Read the model definition and answer for the solid it produces. Units are mm, in the model's axes. Face numbers are marked on the shaded views. A direction names the side the tool comes from. Coordinates: 2 decimals unless noted, no trailing zeros. Order: outer loops, then holes, each group sorted by start corner. A loop starts at its lowest first (then second) coordinate and runs counter-clockwise, first axis right, second up. Notation, with made-up numbers: M 58,75.25 L 88,75.25 A23 cw 88,108.25 Z; hole C -31,61 d3. An arc over 180 degrees is marked long. Use a Markdown table: item, result. Add a question column.
1) For the marked faces 4, 5, 6, 7 and 8, determine the directions among +Z, -Z, +X, -X, +Y, -Y from which every point of the face is accessible in a straight line to the end or side of a thin tool.
2) Find section C-C on z = -30. Write down the section's boundary in (x, y).
3) The mould has two halves that part along Z. Classify the marked faces 1, 2 and 3: released by +Z, released by -Z, zero draft, split by the parting line, or undercut.
4) Find section D-D on z = -46.9. Write down the section's boundary in (x, y), plus the area to 3 significant figures.
5) Each of these flat-tipped pins is pushed along its axis until it touches: pin 1 Ø2.5 at (x, z) = (9.5, -1.5) entering from -Y; pin 2 Ø1.5 at (x, y) = (4.5, -32.5) entering from -Z; pin 3 Ø2.5 at (y, z) = (2.53, -46.9) entering from -X; pin 4 Ø3 at (x, y) = (4, -26) entering from +Z. Where does it stop, or does it pass through?
6) Find section B-B on y = -23. Write down the section's boundary in (x, z), plus the area to 3 significant figures.
7) Find section A-A on z = -60. Write down the section's boundary in (x, y), plus the area to 3 significant figures.
8) Find the intervals of material crossed by probe 1 along Z at (x, y) = (8.5, -32); probe 2 along Z at (x, y) = (8.5, 1); probe 3 along Y at (x, z) = (9.5, -18), in increasing order. Write a range as [from, to].
from build123d import *

# Parameters (mm, degrees)
SKETCH1_W           = 20
SKETCH1_H           = 70
BOSS_EXTRUDE1_DEPTH = 20
SKETCH4_W           = 20
SKETCH4_H           = 70
CUT_EXTRUDE3_DEPTH  = 10
SKETCH5_R           = 6.5
CUT_EXTRUDE4_DEPTH  = 10
SKETCH6_R           = 8.25
CUT_EXTRUDE5_DEPTH  = 4
SKETCH7_R           = 2
CUT_EXTRUDE6_DEPTH  = 20
SKETCH8_R           = 2
CUT_EXTRUDE7_DEPTH  = 20
SKETCH9_W           = 10
SKETCH9_H           = 52
BOSS_EXTRUDE2_DEPTH = 52
SKETCH10_W          = 10
SKETCH10_H          = 52
CUT_EXTRUDE8_DEPTH  = 12
SKETCH11_W          = 42.2
SKETCH11_H          = 42.2
CUT_EXTRUDE9_DEPTH  = 5
SKETCH12_W          = 42.2
SKETCH12_H          = 42.2
CUT_EXTRUDE10_DEPTH = 5
SKETCH13_W          = 52
SKETCH13_H          = 40
BOSS_EXTRUDE3_DEPTH = 10
SKETCH14_R          = 11.5
CUT_EXTRUDE11_DEPTH = 100
SKETCH16_R          = 19
CUT_EXTRUDE12_DEPTH = 100
SKETCH17_R          = 1.5
CUT_EXTRUDE13_DEPTH = 100
CUT_EXTRUDE14_DEPTH = 40
FILLET1_R           = 3
FILLET2_R           = 3
FILLET3_R           = 3
FILLET4_R           = 3
FILLET5_R           = 3
FILLET6_R           = 3
FILLET7_R           = 3
CUT_EXTRUDE15_DEPTH = 2.5
SKETCH21_R          = 3.5
CUT_EXTRUDE16_DEPTH = 13


with BuildPart() as part:
    # Sketch1 → Boss-Extrude1 (new body)
    with BuildSketch(Plane(origin=(0, 0, 0), x_dir=(1, 0, 0), z_dir=(0, 1, 0))):
        with Locations((10, 35)):
            Rectangle(SKETCH1_W, SKETCH1_H)
    extrude(amount=BOSS_EXTRUDE1_DEPTH)

    # Sketch4 → Cut-Extrude3 (cut)
    with BuildSketch(Plane(origin=(0, 20, 0), x_dir=(1, 0, 0), z_dir=(0, 1, 0))):
        with Locations((10, 35)):
            Rectangle(SKETCH4_W, SKETCH4_H)
    extrude(amount=-CUT_EXTRUDE3_DEPTH, mode=Mode.SUBTRACT)

    # Sketch5 → Cut-Extrude4 (cut)
    with BuildSketch(Plane(origin=(0, 10, 0), x_dir=(1, 0, 0), z_dir=(0, 1, 0))):
        with Locations((0, 30)):
            Circle(SKETCH5_R)
    extrude(amount=-CUT_EXTRUDE4_DEPTH, mode=Mode.SUBTRACT)

    # Sketch6 → Cut-Extrude5 (cut)
    with BuildSketch(Plane(origin=(0, 10, 0), x_dir=(1, 0, 0), z_dir=(0, 1, 0))):
        with Locations((0, 30)):
            Circle(SKETCH6_R)
    extrude(amount=-CUT_EXTRUDE5_DEPTH, mode=Mode.SUBTRACT)

    # Sketch7 → Cut-Extrude6 (cut)
    with BuildSketch(Plane(origin=(20, 0, 0), x_dir=(0, 0, -1), z_dir=(1, 0, 0))):
        with Locations((10, 5)):
            Circle(SKETCH7_R)
    extrude(amount=-CUT_EXTRUDE6_DEPTH, mode=Mode.SUBTRACT)

    # Sketch8 → Cut-Extrude7 (cut)
    with BuildSketch(Plane(origin=(0, 10, 0), x_dir=(1, 0, 0), z_dir=(0, 1, 0))):
        with Locations(Location((10, 60, 0), (0, 0, 270))):
            Circle(SKETCH8_R)
    extrude(amount=-CUT_EXTRUDE7_DEPTH, mode=Mode.SUBTRACT)

    # Sketch9 → Boss-Extrude2 (add)
    with BuildSketch(Plane.XZ):
        with Locations((15, -30)):
            Rectangle(SKETCH9_W, SKETCH9_H)
    extrude(amount=BOSS_EXTRUDE2_DEPTH)

    # Sketch10 → Cut-Extrude8 (cut)
    with BuildSketch(Plane.XZ.offset(52)):
        with Locations((15, -30)):
            Rectangle(SKETCH10_W, SKETCH10_H)
    extrude(amount=-CUT_EXTRUDE8_DEPTH, mode=Mode.SUBTRACT)

    # Sketch11 → Cut-Extrude9 (cut)
    with BuildSketch(Plane(origin=(20, 0, 0), x_dir=(0, 0, -1), z_dir=(1, 0, 0))):
        with Locations((30, -14.365359388)):
            Rectangle(SKETCH11_W, SKETCH11_H)
    extrude(amount=-CUT_EXTRUDE9_DEPTH, mode=Mode.SUBTRACT)

    # Sketch12 → Cut-Extrude10 (cut)
    with BuildSketch(Plane(origin=(15, 0, 0), x_dir=(0, 0, -1), z_dir=(1, 0, 0))):
        with Locations((30, -14.365359388)):
            Rectangle(SKETCH12_W, SKETCH12_H)
    extrude(amount=-CUT_EXTRUDE10_DEPTH, mode=Mode.SUBTRACT)

    # Sketch13 → Boss-Extrude3 (add)
    with BuildSketch(Plane.ZY.offset(-10)):
        with Locations((-30, -20)):
            Rectangle(SKETCH13_W, SKETCH13_H)
    extrude(amount=BOSS_EXTRUDE3_DEPTH)

    # Sketch14 → Cut-Extrude11 (cut)
    with BuildSketch(Plane(origin=(0, 0, 0), x_dir=(1, 0, 0), z_dir=(0, 1, 0))):
        with Locations((0, 30)):
            Circle(SKETCH14_R)
    extrude(amount=-CUT_EXTRUDE11_DEPTH, mode=Mode.SUBTRACT)

    # Sketch16 → Cut-Extrude12 (cut)
    with BuildSketch(Plane(origin=(10, 0, 0), x_dir=(0, 0, -1), z_dir=(1, 0, 0))):
        with Locations((30, -14.365359388)):
            Circle(SKETCH16_R)
    extrude(amount=-CUT_EXTRUDE12_DEPTH, mode=Mode.SUBTRACT)

    # Sketch17 → Cut-Extrude13 (cut)
    with BuildSketch(Plane(origin=(10, 0, 0), x_dir=(0, 0, -1), z_dir=(1, 0, 0))):
        with Locations((13.1, 2.534640612)):
            Circle(SKETCH17_R)
        with Locations((46.9, 2.534640612)):
            Circle(SKETCH17_R)
        with Locations((13.1, -31.265359388)):
            Circle(SKETCH17_R)
        with Locations((46.9, -31.265359388)):
            Circle(SKETCH17_R)
    extrude(amount=-CUT_EXTRUDE13_DEPTH, mode=Mode.SUBTRACT)

    # Sketch19 → Cut-Extrude14 (cut)
    with BuildSketch(Plane.XZ.offset(40)):
        Polygon((20, -56), (20, -52), (0, -56), align=None)
        Polygon((20, -4), (20, -8), (0, -4), align=None)
    extrude(amount=-CUT_EXTRUDE14_DEPTH, mode=Mode.SUBTRACT)

    # Fillet1
    fillet1_edges = [part.edges().sort_by_distance(p)[0] for p in [
        (10, -40, -6),
    ]]
    fillet(fillet1_edges, radius=FILLET1_R)

    # Fillet2
    fillet2_edges = [part.edges().sort_by_distance(p)[0] for p in [
        (10, -40, -54),
    ]]
    fillet(fillet2_edges, radius=FILLET2_R)

    # Fillet3
    fillet3_edges = [part.edges().sort_by_distance(p)[0] for p in [
        (10, 0, -54),
    ]]
    fillet(fillet3_edges, radius=FILLET3_R)

    # Fillet4
    fillet4_edges = [part.edges().sort_by_distance(p)[0] for p in [
        (10, 0, -6),
    ]]
    fillet(fillet4_edges, radius=FILLET4_R)

    # Fillet5
    fillet5_edges = [part.edges().sort_by_distance(p)[0] for p in [
        (15, 6.734640612, -51.1),
    ]]
    fillet(fillet5_edges, radius=FILLET5_R)

    # Fillet6
    fillet6_edges = [part.edges().sort_by_distance(p)[0] for p in [
        (15, -35.465359388, -8.9),
    ]]
    fillet(fillet6_edges, radius=FILLET6_R)

    # Fillet7
    fillet7_edges = [part.edges().sort_by_distance(p)[0] for p in [
        (15, -35.465359388, -51.1),
    ]]
    fillet(fillet7_edges, radius=FILLET7_R)

    # Sketch20 → Cut-Extrude15 (cut)
    with BuildSketch(Plane.ZY):
        Polygon((-16.1, -31.265359388), (-14.6, -33.8634356), (-11.6, -33.8634356), (-10.1, -31.265359388), (-11.6, -28.667283177), (-14.6, -28.667283177), align=None)
        Polygon((-49.9, -31.265359388), (-48.4, -33.8634356), (-45.4, -33.8634356), (-43.9, -31.265359388), (-45.4, -28.667283177), (-48.4, -28.667283177), align=None)
        Polygon((-49.9, 2.534640612), (-48.4, -0.0634356), (-45.4, -0.0634356), (-43.9, 2.534640612), (-45.4, 5.132716823), (-48.4, 5.132716823), align=None)
    extrude(amount=-CUT_EXTRUDE15_DEPTH, mode=Mode.SUBTRACT)

    # Sketch21 → Cut-Extrude16 (cut)
    with BuildSketch(Plane(origin=(20, 0, 0), x_dir=(0, 0, -1), z_dir=(1, 0, 0))):
        with Locations((10, 5)):
            Circle(SKETCH21_R)
    extrude(amount=-CUT_EXTRUDE16_DEPTH, mode=Mode.SUBTRACT)


solid = part.part
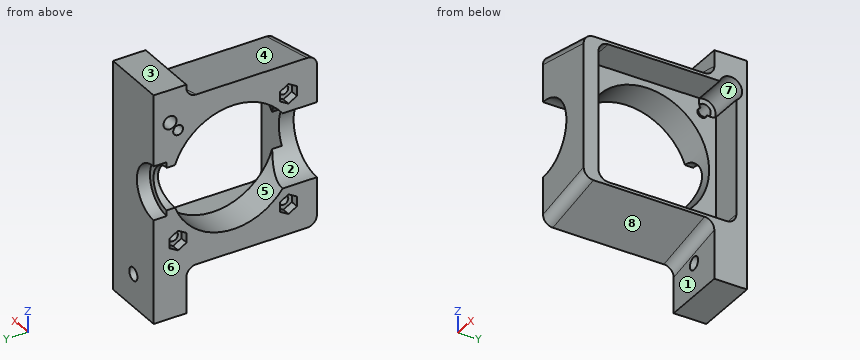
Check result:
| question | item | result |
|---|---|---|
| 1 | face 4 | +Z, +X, -Y |
| 1 | face 5 | +X, -X |
| 1 | face 6 | +Z, -Z, -X, +Y, -Y |
| 1 | face 7 | +X |
| 1 | face 8 | -Z, +X, -Y |
| 2 | outline | M 6.5,4.63 L 10,4.63 L 10,6.73 L 20,6.73 L 20,10 L 8.25,10 L 8.25,6 L 6.5,6 Z; M 11.5,-40 L 20,-40 L 20,-35.47 L 11.5,-35.47 Z |
| 3 | face 1 | zero draft |
| 3 | face 2 | undercut |
| 3 | face 3 | released by +Z |
| 4 | outline | M 0,-40 L 20,-40 L 20,-35.47 L 10,-35.47 L 10,-32.77 L 2.5,-32.77 L 2.5,-33.86 L 0,-33.86 Z; M 0,-28.67 L 2.5,-28.67 L 2.5,-29.77 L 10,-29.77 L 10,-23.05 L 0,-23.05 Z; M 0,-5.68 L 10,-5.68 L 10,1.03 L 2.5,1.03 L 2.5,-0.06 L 0,-0.06 Z; M 0,5.13 L 2.5,5.13 L 2.5,4.03 L 10,4.03 L 10,6.73 L 20,6.73 L 20,10 L 0,10 Z |
| 4 | area | 333 mm2 |
| 5 | pin 1 | stops at y = 0 |
| 5 | pin 2 | stops at z = -55.25 |
| 5 | pin 3 | passes through |
| 5 | pin 4 | stops at z = -4.5 |
| 6 | outline | M 0,-56 L 20,-52 L 20,-51.1 L 10,-51.1 L 10,-46.92 L 0,-46.92 Z; M 0,-13.08 L 10,-13.08 L 10,-8.9 L 20,-8.9 L 20,-8 L 0,-4 Z |
| 6 | area | 200 mm2 |
| 7 | outline | M 0,0 L 8,0 L 8,10 L 0,10 Z; M 12,0 L 20,0 L 20,10 L 12,10 Z |
| 7 | area | 160 mm2 |
| 8 | probe 1 | z = [-54.3, -48.21], [-45.59, -37.75], [-22.25, -14.41], [-11.79, -5.7] |
| 8 | probe 2 | z = [-70, -61.32], [-58.68, -41.18], [-18.82, 0] |
| 8 | probe 3 | y = [-40, -29.1], [0.37, 10] |
